The figure shows three views and two pictorial views of one solid part (mm, origin at its lowest corner). Answer the questions. Round coordinates to 2 decimals unless told otherwise and drop trailing zeros. Write each loop counter-clockwise with the first axis right and the second up, starting at its lowest first coordinate (ties: lowest second). Pieces come first, ordered by that corner, then holes.
Item 1: Each of these flat-tipped pins is pushed along its axis until it touches: pin 1 (1.7 mm diameter, centred on x = 26.5, z = 36.5, fed in from -Y); pin 2 (5 mm diameter, centred on x = 62, y = 6.5, fed in from -Z); pin 3 (6.5 mm diameter, centred on x = 105, z = 37.5, fed in from -Y). Where does it stop, or does it pass through?
Item 2: Find the intervals of material crossed by probe 1 along Z at (x, y) = (122, 3.5); probe 2 along X at (y, z) = (5.25, 67); probe 3 along X at (y, z) = (0.75, 60.5), in increasing order.
Item 3: Find section B-B on z = 9. Give the vertices of the cut face in (x, y).
Item 4: Find section A-A on x = 10. Give the vertices of the cut face in (y, z), then the cut area to 3 significant figures.
Item 5: Find section C-C on z = 35. Give the vertices of the cut face in (x, y), then the cut area to 3 significant figures.
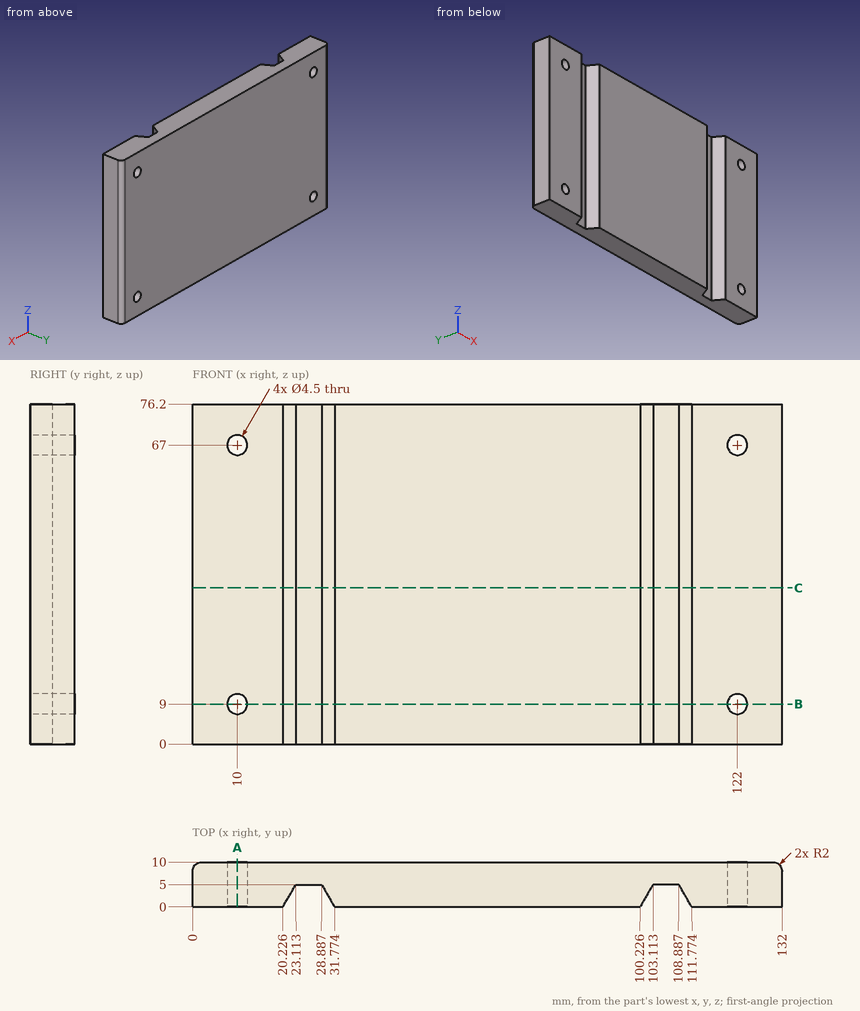
Check values:
1. pin 1: stops at y = 5
1. pin 2: stops at z = 0
1. pin 3: stops at y = 2.64
2. probe 1: z = 0 to 6.75, 11.25 to 64.75, 69.25 to 76.2
2. probe 2: x = 0 to 7.75, 12.25 to 119.75, 124.25 to 132
2. probe 3: x = 0 to 20.66, 31.34 to 100.66, 111.34 to 132
3. outline: (0, 0) - (7.75, 0) - (7.75, 10) - (2, 10) arc R2 ccw to (0, 8) - close; (12.25, 0) - (20.23, 0) - (23.11, 5) - (28.89, 5) - (31.77, 0) - (100.23, 0) - (103.11, 5) - (108.89, 5) - (111.77, 0) - (119.75, 0) - (119.75, 10) - (12.25, 10) - close; (124.25, 0) - (132, 0) - (132, 8) arc R2 ccw to (130, 10) - (124.25, 10) - close
4. outline: (0, 0) - (10, 0) - (10, 6.75) - (0, 6.75) - close; (0, 11.25) - (10, 11.25) - (10, 64.75) - (0, 64.75) - close; (0, 69.25) - (10, 69.25) - (10, 76.2) - (0, 76.2) - close
4. area: 672 mm2
5. outline: (0, 0) - (20.23, 0) - (23.11, 5) - (28.89, 5) - (31.77, 0) - (100.23, 0) - (103.11, 5) - (108.89, 5) - (111.77, 0) - (132, 0) - (132, 8) arc R2 ccw to (130, 10) - (2, 10) arc R2 ccw to (0, 8) - close
5. area: 1,230 mm2
